Geometry: see drawing. Coordinates: mm, zero at the bounding-box minimum. A direction names the side the tool comes from. Round coordinates to 2 decimals unless told otherwise and drop trailing zeros. Order: outer loops, then holes, each group sorted by start corner. A loop starts at its lowest first (then second) coordinate and runs counter-clockwise, first axis right, second up. Notation, with made-up numbers: (1.5, 57) - (31.5, 57) arc R18 ccw to (31.5, 91) - close; hole circle Ø9 at (45, 8). An arc over 180 degrees is marked (long way). Put each result on its own line as item: value. Start each with the question number.
1) Mould query, pull axis Y, two halves, no side actions, for the marked faces 4, 5, 6 and 7. Classes: +Y half, -Y half, draft (parallel to the pull), parting line (faces both ways), or undercut.
2) Section D-D on x = 54. Output: boundary loops of the cut face in (y, z), then the cut area to 3 significant figures.
3) Section A-A on y = 6. Output: boundary loops of the cut face in (x, z).
4) Access query for the marked faces 1, 2 and 3. Directions: +Z, -Z, +X, -X, +Y, -Y. A direction counts if a zero-diameter tool reaches every point of the face in a straight line with its end or side. Return the directions, or none.
5) Section B-B on x = 6. Output: boundary loops of the cut face in (y, z).
6) Contact query for flat-ended pins moving along their axis: P1, Ø6, axis at x = 35.5, z = 2, coming from the -Y side; P2, Ø5, axis at x = 16, z = 5.5, coming from the +Y side; P3, Ø5, axis at y = 10.5, z = 7.5, coming from the +X side. Output: stop coordinate, or through.
7) Section C-C on z = 1. Output: boundary loops of the cut face in (x, y).
8) Line query: probe 1 along X at (y, z) = (5.75, 3.25) (1 decimal); probe 2 along Y at (x, z) = (6, 5.25); probe 3 along X at (y, z) = (7.25, 6). Output: solid intervals per line, ascending. Write a range as [from, to].
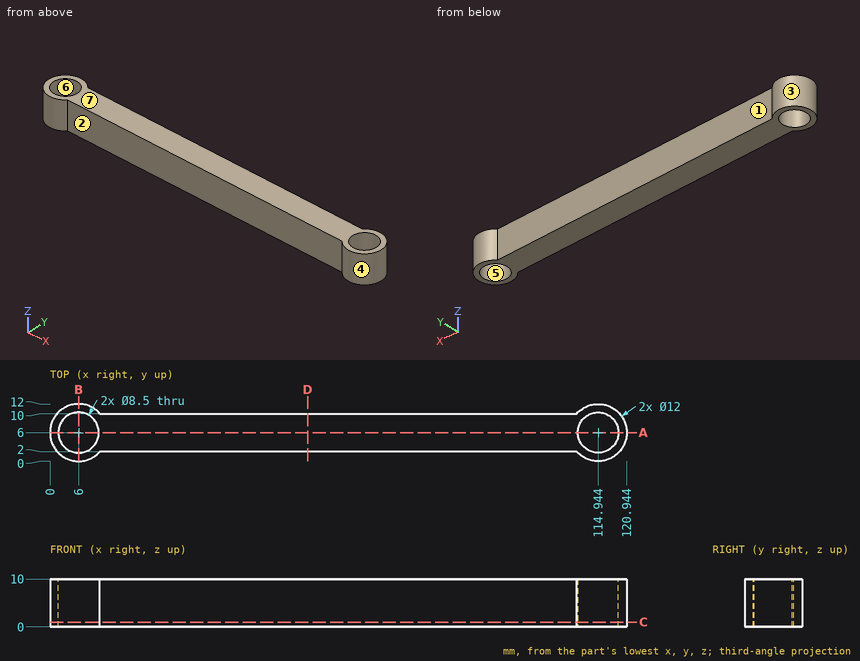
Answer sheet:
1. face 4: parting line
1. face 5: undercut
1. face 6: undercut
1. face 7: draft
2. outline: (2, 0) - (10, 0) - (10, 10) - (2, 10) - close
2. area: 80.0 mm^2
3. outline: (0, 0) - (1.75, 0) - (1.75, 10) - (0, 10) - close; (10.25, 0) - (110.69, 0) - (110.69, 10) - (10.25, 10) - close; (119.19, 0) - (120.94, 0) - (120.94, 10) - (119.19, 10) - close
4. face 1: +Z, -Z, +Y
4. face 2: +Z, -Z, -Y
4. face 3: +Z, -Z
5. outline: (0, 0) - (1.75, 0) - (1.75, 10) - (0, 10) - close; (10.25, 0) - (12, 0) - (12, 10) - (10.25, 10) - close
6. P1: y = 2
6. P2: y = 10
6. P3: x = 120.6
7. outline: (10.47, 2) - (110.47, 2) arc R6 ccw (long way) to (110.47, 10) - (10.47, 10) arc R6 ccw (long way) to start; hole circle Ø8.5 at (6, 6); hole circle Ø8.5 at (114.94, 6)
8. probe 1: [0, 1.8], [10.2, 110.7], [119.2, 120.9]
8. probe 2: [0, 1.75], [10.25, 12]
8. probe 3: [0.13, 1.94], [10.06, 110.88], [119.01, 120.81]
